Part model, mm, in its own coordinate system. Face numbers are marked on the shaded views. Round coordinates to 2 decimals unless told otherwise and drop trailing zeros. Write each loop counter-clockwise with the first axis right and the second up, starting at its lowest first coordinate (ties: lowest second). Pieces come first, ordered by that corner, then holes. Notation, with made-up numbers: (54.25, 78.25) -> (91.25, 78.25) arc R25 cw to (91.25, 115.25) -> close; hole circle Ø1 at (45, 88). An arc over 180 degrees is marked (long way). Return JSON: item names as keys, results as strings. Group by question number.
```python
from build123d import *

# Parameters (mm, degrees)
F0_R     = 12.7
F1_DEPTH = 152.4
F2_W     = 127
F2_H     = 127
F3_DEPTH = 53.830817


with BuildPart() as f1:
    # F0 (on Top) → F1 (new body)
    with BuildSketch(Plane.XY):
        Circle(F0_R)
    extrude(amount=F1_DEPTH)


with BuildPart() as f3:
    # F2 (on Top) → F3 (new body)
    with BuildSketch(Plane.XY):
        Rectangle(F2_W, F2_H)
    extrude(amount=F3_DEPTH)

    # F4: cut F1
    add(f1.part, mode=Mode.SUBTRACT)


solid = f3.part
```
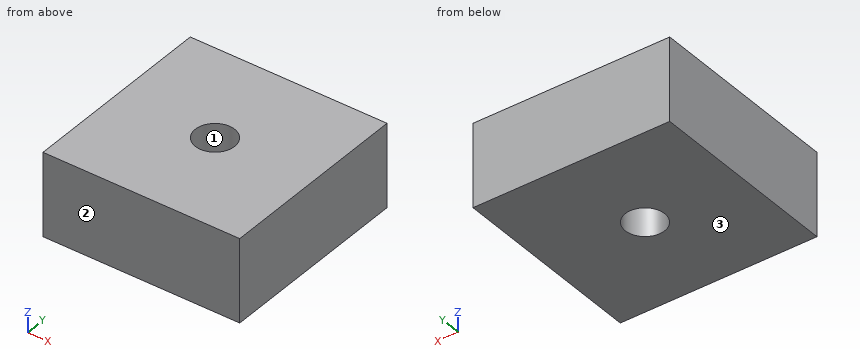
Item 1: Flat gauge pin, fed straight in: P1, Ø10, axis at x = -41.5, y = 25.5, coming from the -Z side. Where does the tip first touch, or does it go through?
Item 2: Wall check: L1, parallel to X at y = 0, z = 20; L2, parallel to X at y = 8.5, z = 16. Give the ranges that are in metal, low to high.
Item 3: Cut at C-C (z = 46.5). Write the cut outline in (x, y).
Item 4: Two-plate mould, pull along Y, no slides. Class the marked faces 1, 2 and 3: released by +Y, released by -Y, zero draft, split by the parting line, or undercut.
Item 5: Cut at A-A (y = 0). Write the cut outline in (x, z).
Checks:
{
 "1": {"P1": "stops at z = 0"},
 "2": {"L1": "x = -63.5 to -12.7, 12.7 to 63.5", "L2": "x = -63.5 to -9.44, 9.44 to 63.5"},
 "3": {"outline": "(-63.5, -63.5) -> (63.5, -63.5) -> (63.5, 63.5) -> (-63.5, 63.5) -> close; hole circle Ø25.4 at (0, 0)"},
 "4": {"face 1": "undercut", "face 2": "released by -Y", "face 3": "zero draft"},
 "5": {"outline": "(-63.5, 0) -> (-12.7, 0) -> (-12.7, 53.83) -> (-63.5, 53.83) -> close; (12.7, 0) -> (63.5, 0) -> (63.5, 53.83) -> (12.7, 53.83) -> close"}
}
